Could you check a few things on this model? Use its own coordinates, in mm. A direction names the side the tool comes from. Give positions to 0.01 mm unless a question says otherwise; leave off trailing zeros. Loops run counter-clockwise (first coordinate to the right, second up) from the corner with the lowest first, then second, coordinate; pieces in that order, holes last. Notation, with made-up numbers: (2.5, 41) -> (47.5, 41) arc R7 cw to (47.5, 49) -> close; hole circle Ø8 at (19.5, -1.5). An arc over 180 degrees is marked (long way). Write each question's results on one line, items separated by ' | '. Start each with the question number.
Q1. We'd pull the mould along Y, two halves only. Please class faces 1 (the face through (2, -21.5, 0)), 2 (the face through (125, -1, -6.5)), 3 (the face through (85, 0, -56)), 4 (the face through (9, -10, -2)): released by +Y, released by -Y, zero draft, split by the parting line, or undercut.
Q2. If we section it at C-C, the plane z = -62: List the corners of the cut face in (x, y) for me, plus the area to 3 significant figures.
Q3. If I drill on line 1 along Z through (x, y) = (137.5, -1.5); line 2 along Y through (x, z) = (21, -5.5); line 3 along X through (y, z) = (-2, -11.5), over which ranges is the centre line in solid material (lowest first)?
Q4. If we section it at B-B, the plane y = -10: List the corners of the cut face in (x, z) for me.
Q5. Will these pins go through, and if not, where does the flat tip stop? P1, Ø12, axis at x = 53, z = -9, coming from the -Y side; P2, Ø2.5, axis at y = -2, z = -28.5, coming from the -X side; P3, Ø1.6, axis at x = 168, y = -21, coming from the -Z side; P4, Ø5.5, axis at x = 12, y = -15, coming from the -Z side.
Q6. If we section it at D-D, the plane x = 12: List the corners of the cut face in (y, z) for me, plus the area to 3 significant figures.
Q7. If we section it at A-A, the plane x = 73.5: List the corners of the cut face in (y, z) for me, plus the area to 3 significant figures.
Q8. Which directions (+Z, -Z, +X, -X, +Y, -Y) give clear straight access to the entire face, cutting with the end or side of a thin tool? Please do faces 5 (the face through (45, -1, -56.5)), 6 (the face through (167, -21.5, 0)), 7 (the face through (155.6, -12.1, 0.5)).
from build123d import *

# Parameters (mm, degrees)
F0_W          = 170
F0_H          = 66
F0_R          = 2.38125
F1_DEPTH      = 3
F0_H_2        = 1.5
F2_DEPTH      = 21.5
F3_W          = 170
F3_H          = 2
F4_DEPTH      = 2
F5_W          = 160
F5_H          = 18.5
F6_DEPTH      = 3.501
F8_DEPTH      = 3
F8_DEPTH_BACK = 2


with BuildPart() as f1:
    # F0 (on Front) → F1 (new body)
    with BuildSketch(Plane.XZ):
        with Locations((85, -34.5)):
            Rectangle(F0_W, F0_H)
        with Locations((5, -62)):
            Circle(F0_R, mode=Mode.SUBTRACT)
        with Locations((165, -62)):
            Circle(F0_R, mode=Mode.SUBTRACT)
        Polygon((5, -56.5), (5, -6.5), (83, -6.5), (85, -8.5), (87, -6.5), (165, -6.5), (165, -56.5), (87, -56.5), (85, -54.5), (83, -56.5), align=None, mode=Mode.SUBTRACT)
    extrude(amount=F1_DEPTH)

    # F0 (on Front) → F2 (join)
    with BuildSketch(Plane.XZ):
        with Locations((85, -0.75)):
            Rectangle(F0_W, F0_H_2)
    extrude(amount=F2_DEPTH)

    # F3 (on face) → F4 (join)
    with BuildSketch(Plane(origin=(0, 0, -1.5), x_dir=(1, 0, 0), z_dir=(0, 0, -1))):
        with Locations((85, 20.5)):
            Rectangle(F3_W, F3_H)
    extrude(amount=F4_DEPTH)

    # F5 (on face) → F6 (cut, through all)
    with BuildSketch(Plane(origin=(0, 0, -3.5), x_dir=(1, 0, 0), z_dir=(0, 0, -1))):
        with Locations((85, 12.25)):
            Rectangle(F5_W, F5_H)
    extrude(amount=-F6_DEPTH, mode=Mode.SUBTRACT)

    # F7 (on face) → F8 (join, two sides)
    with BuildSketch(Plane.XY) as f8_sk:
        Polygon((0, 0), (0, -21.5), (5, -21.5), (23.5, -3), (146.5, -3), (165, -21.5), (170, -21.5), (170, 0), align=None)
    extrude(amount=F8_DEPTH)
    extrude(f8_sk.sketch, amount=-F8_DEPTH_BACK)


solid = f1.part
Final values:
1) face 1: released by -Y | face 2: zero draft | face 3: released by +Y | face 4: undercut
2) outline: (0, -3) -> (2.62, -3) -> (2.62, 0) -> (0, 0) -> close; (7.38, -3) -> (162.62, -3) -> (162.62, 0) -> (7.38, 0) -> close; (167.38, -3) -> (170, -3) -> (170, 0) -> (167.38, 0) -> close | area: 481 mm²
3) line 1: z = -67.5 to -56.5, -6.5 to 3 | line 2: y = -3 to 0 | line 3: x = 0 to 5, 165 to 170
4) outline: (0, -2) -> (16.5, -2) -> (16.5, 3) -> (0, 3) -> close; (153.5, -2) -> (170, -2) -> (170, 3) -> (153.5, 3) -> close
5) P1: stops at y = -3 | P2: stops at x = 0 | P3: stops at z = -3.5 | P4: stops at z = -2
6) outline: (-14.5, -2) -> (-3, -2) -> (-3, -6.5) -> (0, -6.5) -> (0, 3) -> (-14.5, 3) -> close; (-3, -67.5) -> (0, -67.5) -> (0, -56.5) -> (-3, -56.5) -> close | area: 119 mm²
7) outline: (-3, -67.5) -> (0, -67.5) -> (0, -56.5) -> (-3, -56.5) -> close; (-3, -6.5) -> (0, -6.5) -> (0, 3) -> (-3, 3) -> close | area: 61.5 mm²
8) face 5: +Y, -Y | face 6: +Z, -Z, +X, -X, -Y | face 7: +Z, -Z, -Y
